Geometry check sheet. Reference: drawing and pictorial views, mm from the part's lowest x, y, z. A direction names the side the tool comes from. Give positions to 0.01 mm unless a question says otherwise; leave off trailing zeros. Loops run counter-clockwise (first coordinate to the right, second up) from the corner with the lowest first, then second, coordinate; pieces in that order, holes last. Notation, with made-up numbers: (-38.75, 58.25) - (-3.75, 58.25) arc R26 cw to (-3.75, 76.25) - close; hole circle Ø8 at (4.5, -9). An arc over 180 degrees is marked (long way). One line per question, with ' | ' between items. Start each with the question number.
1. Mould release check, pull along X, two halves, no side actions. Record for the marked faces 3, 4 and 5: +X half, -X half, draft (parallel to the pull), parting line (faces both ways), or undercut.
2. Section check A-A, the plane x = 8.5. Enter the section's corners in (y, z), then the cut area to 3 significant figures.
3. Thickness scan on line 1 along Z through (x, y) = (8, 1.75); line 2 along Y through (x, z) = (10.75, 10.25); line 3 along Y through (x, z) = (14.5, 14). Record the ranges inside material, lowest first. Write a range as from..to.
4. Section check C-C, the plane z = 8.5. Enter the section's corners in (x, y).
5. Depth check by flat-ended pin: pin 1 Ø1 at (x, y) = (8.5, 3) entering from -Z; pin 2 Ø4 at (x, z) = (8.5, 4.5) entering from +Y; pin 3 Ø1.5 at (x, y) = (15, 2) entering from +Z. Enter the tip coordinate at first touch or a pass-through.
6. Tool access check on the marked faces 1 and 2. Record the directions out of +Z, -Z, +X, -X, +Y, -Y that give a thin tool (end or side, any length) a straight path to the whole face; none if there is none.
7. Section check B-B, the plane z = 4.5. Enter the section's corners in (x, y).
8. Section check D-D, the plane y = 4.3. Enter the section's corners in (x, z), then the cut area to 3 significant figures.
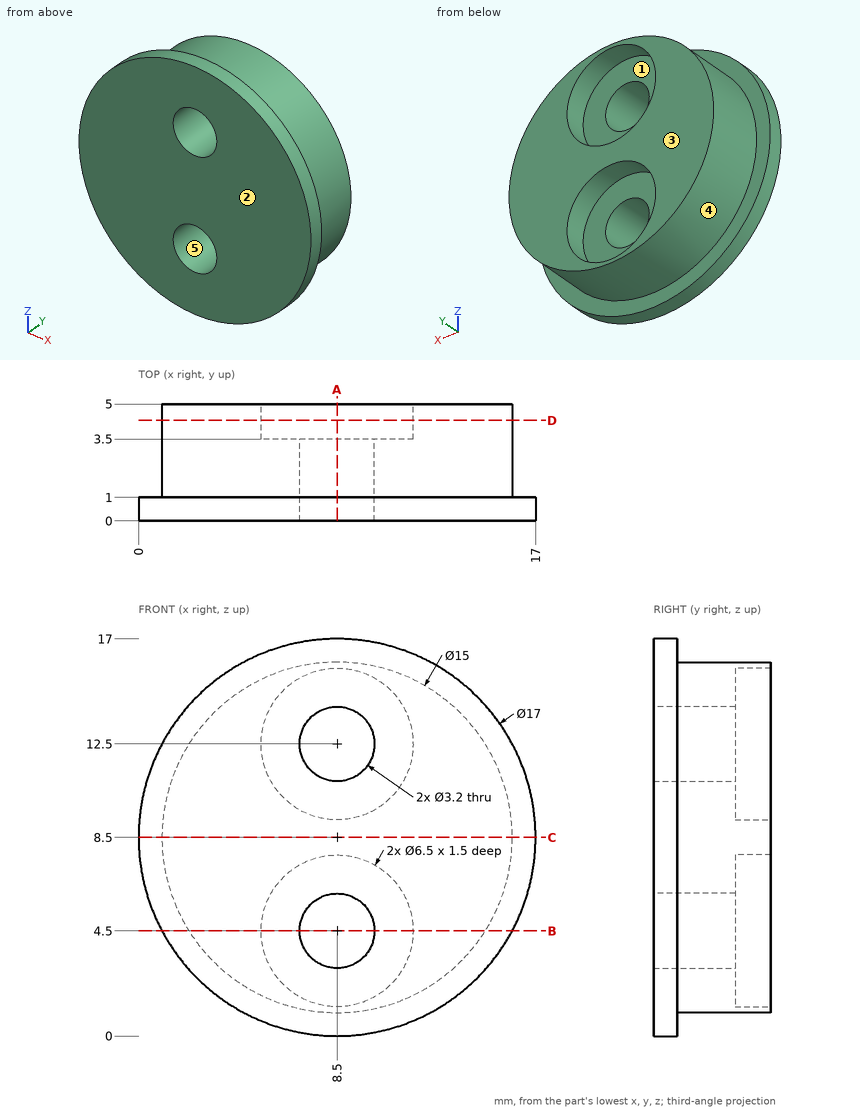
Results list:
1) face 3: draft | face 4: parting line | face 5: undercut
2) outline: (0, 0) - (1, 0) - (1, 1) - (5, 1) - (5, 1.25) - (3.5, 1.25) - (3.5, 2.9) - (0, 2.9) - close; (0, 6.1) - (3.5, 6.1) - (3.5, 7.75) - (5, 7.75) - (5, 9.25) - (3.5, 9.25) - (3.5, 10.9) - (0, 10.9) - close; (0, 14.1) - (3.5, 14.1) - (3.5, 15.75) - (5, 15.75) - (5, 16) - (1, 16) - (1, 17) - (0, 17) - close | area: 35.1 mm²
3) line 1: 1.02..2.98, 6.02..10.98, 14.02..15.98 | line 2: 0..3.5 | line 3: 0..1
4) outline: (0, 0) - (17, 0) - (17, 1) - (16, 1) - (16, 5) - (1, 5) - (1, 1) - (0, 1) - close
5) pin 1: z = 1 | pin 2: y = 3.5 | pin 3: z = 13.32
6) face 1: +Y | face 2: +Z, -Z, +X, -X, -Y
7) outline: (1, 0) - (6.9, 0) - (6.9, 3.5) - (5.25, 3.5) - (5.25, 5) - (2.16, 5) - (2.16, 1) - (1, 1) - close; (10.1, 0) - (16, 0) - (16, 1) - (14.84, 1) - (14.84, 5) - (11.75, 5) - (11.75, 3.5) - (10.1, 3.5) - close
8) outline: circle Ø15 at (8.5, 8.5); hole circle Ø6.5 at (8.5, 4.5); hole circle Ø6.5 at (8.5, 12.5) | area: 110 mm²
